Work out the finished part from the listing and answer in its coordinate system (mm). Face numbers are marked on the shaded views. A direction names the side the tool comes from. Coordinates: 2 decimals unless noted, no trailing zeros. Loops run counter-clockwise (first coordinate to the right, second up) from the corner with the lowest first, then second, coordinate; pieces in that order, holes last. Notation, with made-up numbers: (-35, 56) - (-19, 56) arc R20 ccw to (-19, 70) - close; hole circle Ø2 at (-22, -0.75). An arc over 180 degrees is marked (long way). Write each question's results on one line, items separated by ' | '. Start each with the question number.
1. Determine the mould class of the marked faces 1, 2 and 3 for opening direction Y: released by +Y, released by -Y, zero draft, split by the parting line, or undercut.
2. Which of the six approach directions +Z, -Z, +X, -X, +Y, -Y give full straight-line access (tool end or side, diameter ignored) to the marked faces 4, 5 and 6?
3. Find the intervals of material crossed by line 1 along Y through (x, z) = (0.15, 0); line 2 along Y through (x, z) = (1.65, 0); line 3 along X through (y, z) = (-3, -1.25), in increasing order. Write a range as [from, to].
4. Each of these flat-tipped pins is pushed along its axis until it touches: P1, Ø1, axis at x = 2, y = 2, coming from the +Z side; P2, Ø1.5, axis at x = 2, y = -2, coming from the +Z side. Where does it stop, or does it pass through?
5. A cutting plane is placed at A-A on z = 0. Determine the outline of the cut face in (x, y).
6. A cutting plane is placed at C-C on x = 2.4. Determine the outline of the cut face in (y, z), then the cut area to 3 significant figures.
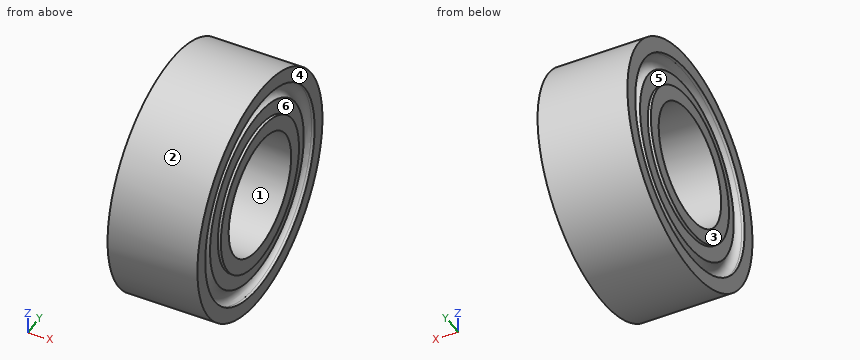
from build123d import *


with BuildPart() as part:
    # 草图1 → 旋转1 (revolve)
    with BuildSketch(Plane.XY, mode=Mode.PRIVATE) as revolve_1_sk:
        with BuildLine():
            Line((0.1, 3.5), (0, 3.5))
            Line((0, 3.5), (0, 4))
            Line((0, 4), (3, 4))
            Line((3, 4), (3, 3.5))
            Line((3, 3.5), (2.9, 3.5))
            ThreePointArc((2.9, 3.5), (2.65, 3.25), (2.9, 3))
            Line((2.9, 3), (2.9, 2.5))
            Line((2.9, 2.5), (3, 2.5))
            Line((3, 2.5), (3, 2))
            Line((3, 2), (0, 2))
            Line((0, 2), (0, 2.5))
            Line((0, 2.5), (0.1, 2.5))
            Line((0.1, 2.5), (0.1, 3))
            ThreePointArc((0.1, 3), (0.35, 3.25), (0.1, 3.5))
        make_face()
    revolve(revolve_1_sk.sketch.rotate(Axis((0, 0, 0), (1, 0, 0)), 90), axis=Axis((0, 0, 0), (1, 0, 0)))


solid = part.part
Values:
1) face 1: undercut | face 2: split by the parting line | face 3: zero draft
2) face 4: +Z, -Z, +X, +Y, -Y | face 5: -X | face 6: +X
3) line 1: [-4, -3.49], [-3.01, -2], [2, 3.01], [3.49, 4] | line 2: [-4, -2], [2, 4] | line 3: [0.35, 2.65]
4) P1: z = 3.71 | P2: z = 3.8
5) outline: (0, -4) - (3, -4) - (3, -3.5) - (2.9, -3.5) arc R0.25 cw to (2.9, -3) - (2.9, -2.5) - (3, -2.5) - (3, -2) - (0, -2) - (0, -2.5) - (0.1, -2.5) - (0.1, -3) arc R0.25 cw to (0.1, -3.5) - (0, -3.5) - close; (0, 2) - (3, 2) - (3, 2.5) - (2.9, 2.5) - (2.9, 3) arc R0.25 cw to (2.9, 3.5) - (3, 3.5) - (3, 4) - (0, 4) - (0, 3.5) - (0.1, 3.5) arc R0.25 cw to (0.1, 3) - (0.1, 2.5) - (0, 2.5) - close
6) outline: circle Ø8 at (0, 0); hole circle Ø4 at (0, 0) | area: 37.7 mm^2
